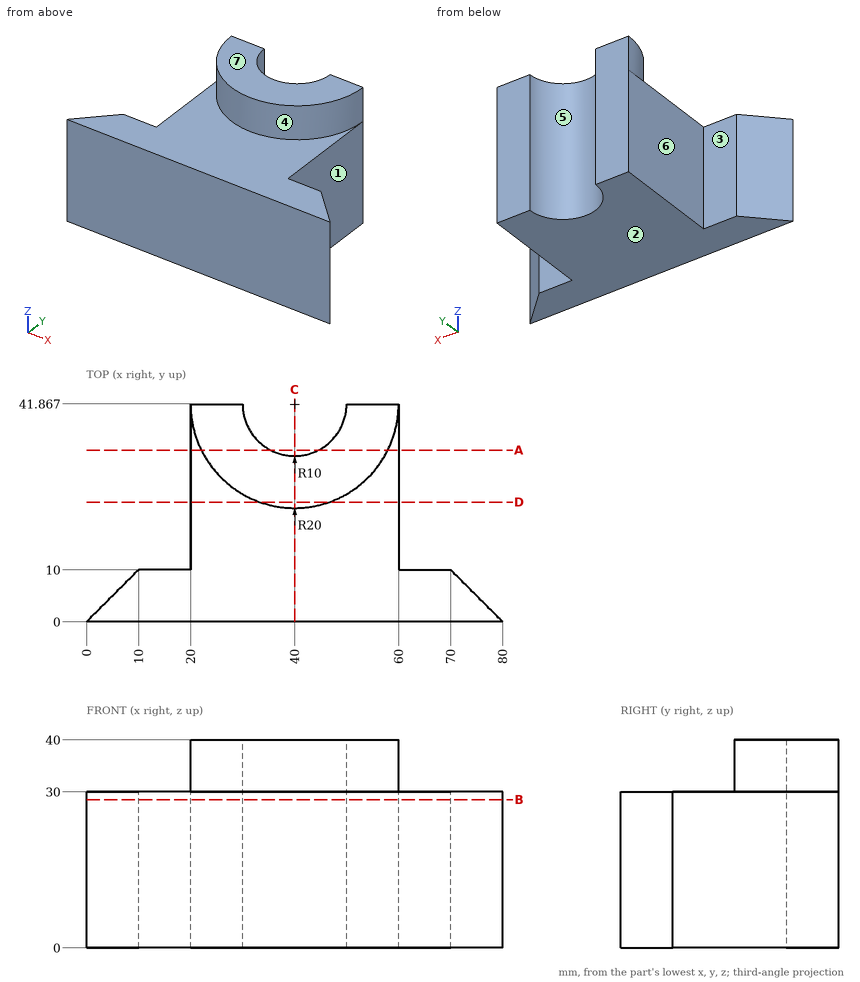
Study the drawing (mm; zero at the part's minimum x, y, z) and answer. A direction names the side the tool comes from. Give positions to 0.01 mm unless a question says otherwise; leave off trailing zeros. Write each loop counter-clockwise with the first axis right and the second up, starting at its lowest first coordinate (ties: lowest second). Pieces come first, ordered by that corner, then holes. Notation, with made-up numbers: (9.25, 53) -> (58.25, 53) arc R16 ccw to (58.25, 84) -> close; hole circle Ø2 at (44.25, 47). An arc over 180 degrees is marked (long way). Answer in a Markdown table with one row per item.
1) Section C-C on x = 40 is taken. Give the vertices of the cut face in (y, z), plus the area to 3 significant figures.
Results list:
| item | result |
|---|---|
| outline | (0, 0) -> (31.87, 0) -> (31.87, 40) -> (21.87, 40) -> (21.87, 30) -> (0, 30) -> close |
| area | 1,060 mm^2 |
2) Section D-D on y = 23 is taken. Give the vertices of the cut face in (x, z), plus the area to 3 significant figures.
Results list:
| item | result |
|---|---|
| outline | (20, 0) -> (60, 0) -> (60, 30) -> (46.64, 30) -> (46.64, 40) -> (33.36, 40) -> (33.36, 30) -> (20, 30) -> close |
| area | 1,330 mm^2 |
3) Determine the mould class of the marked faces 5, 6 and 7 for opening direction X: released by +X, released by -X, zero draft, split by the parting line, or undercut.
Results list:
| item | result |
|---|---|
| face 5 | undercut |
| face 6 | released by -X |
| face 7 | zero draft |
4) Straight lines are drawn through the part: line 1 (X direction, y = 25, z = 2); line 2 (Z direction, x = 56.5, y = 25); line 3 (X direction, y = 33, z = 16) (1 decimal). For each, find the intervals that lie inside material, in ascending order. Write a range as [from, to].
Results list:
| item | result |
|---|---|
| line 1 | [20, 60] |
| line 2 | [0, 30] |
| line 3 | [20, 35.4], [44.6, 60] |
5) Section A-A on y = 33 is taken. Give the vertices of the cut face in (x, z).
Results list:
| item | result |
|---|---|
| outline | (20, 0) -> (35.38, 0) -> (35.38, 40) -> (22.07, 40) -> (22.07, 30) -> (20, 30) -> close; (44.62, 0) -> (60, 0) -> (60, 30) -> (57.93, 30) -> (57.93, 40) -> (44.62, 40) -> close |
6) Section B-B on z = 28.5 is taken. Give the vertices of the cut face in (x, y).
Results list:
| item | result |
|---|---|
| outline | (0, 0) -> (80, 0) -> (70, 10) -> (60, 10) -> (60, 41.87) -> (50, 41.87) arc R10 cw to (30, 41.87) -> (20, 41.87) -> (20, 10) -> (10, 10) -> close |
7) A tool of negligible diameter and unlimited length cuts with its end or side. For the marked faces 1, 2, 3 and 4, from which of +Z, -Z, +X, -X, +Y, -Y can it reach the whole face along a straight path? Write none if from no direction.
Results list:
| item | result |
|---|---|
| face 1 | +Z, -Z, +X, +Y |
| face 2 | -Z, +X, -X, +Y, -Y |
| face 3 | +Z, -Z, -X, +Y |
| face 4 | +Z, -Y |
8) Each of these flat-tipped pins is pushed along its axis until it touches: pin 1 Ø4 at (x, y) = (37, 10) entering from +Z; pin 2 Ø1.5 at (y, z) = (8, 10.5) entering from +X; pin 3 Ø3 at (x, z) = (66.5, 18) entering from +Y; pin 4 Ø1.5 at (x, z) = (26, 11.5) entering from -Y. Where does it stop, or does it pass through?
Results list:
| item | result |
|---|---|
| pin 1 | z = 30 |
| pin 2 | x = 72.75 |
| pin 3 | y = 10 |
| pin 4 | y = 0 |
